Source: CAD feature listing. Evaluate the final solid. Frame: model axes, mm. A direction names the side the tool comes from. Round coordinates to 2 decimals unless told otherwise and drop trailing zeros. Order: outer loops, then holes, each group sorted by start corner. A loop starts at its lowest first (then second) coordinate and runs counter-clockwise, first axis right, second up. Notation, with made-up numbers: (15, 3) - (21, 3) arc R30 ccw to (21, 38) - close; hole circle Ø5 at (-14, -16). An arc over 180 degrees is marked (long way). Return JSON: item names as keys, results as strings. Group by question number.
1) Access query for faces 1 (the flat face through (6, -4, 60)), 2 (the flat face through (7.5, 0, 17)), 3 (the flat face through (-5, 1.1, 39)), 4 (the flat face through (6, -4, 19)), 5 (the flat face through (-6, 4, 39)). Directions: +Z, -Z, +X, -X, +Y, -Y. A direction counts if a zero-diameter tool reaches every point of the face in a straight line with its end or side. Return the directions, or none.
2) Section A-A, the plane y = -5. Return loops of the section in (x, z).
3) Section C-C, the plane y = 0.25. Return loops of the section in (x, z), plus the area to 3 significant figures.
4) Ray query, line 1 (X direction, y = -2.5, z = 72); line 2 (X direction, y = 0, z = 44); line 3 (Z direction, x = 10.25, y = 1.25). Return the intervals inside material, ascending. Write a range as from..to.
5) Section B-B, the plane z = 63. Return loops of the section in (x, y), plus the area to 3 significant figures.
6) Contact query for flat-ended pins moving along their axis: P1, Ø0.9, axis at x = 6, z = 51.5, coming from the -Y side; P2, Ø5, axis at y = 2.5, z = 35, coming from the +X side; P3, Ø1.8, axis at x = 5, z = 35.5, coming from the +Y side. Output: stop coordinate, or through.
7) Section D-D, the plane x = -0.75. Return loops of the section in (y, z), plus the area to 3 significant figures.
8) Mould query, pull axis X, two halves, no side actions, for faces 6 (the flat face through (4.5, 3, 39)), 7 (the flat face through (-6, -4, 39)), 8 (the flat face through (7.5, 0, 61)). Classes: pulls with the +X half, pulls with the -X half, needs draft (parallel to the pull), parting line crosses it, or undercut.
Autodesk Inventor part; units mm, degrees
ref_plane "YZ Plane" through (0, 0, 0) normal (1, 0, 0) x (0, 1, 0)
ref_plane "XZ Plane" through (0, 0, 0) normal (0, 1, 0) x (-1, 0, 0)
ref_plane "XY Plane" through (0, 0, 0) normal (0, 0, 1) x (1, 0, 0)
sketch "Sketch1" plane through (0, 0, 0) normal (0, 0, 1) x (1, 0, 0)
  line L0 (-7.5, 7.5) -> (7.5, 7.5)
  line L1 (7.5, 7.5) -> (7.5, -7.5)
  line L2 (7.5, -7.5) -> (-7.5, -7.5)
  line L3 (-7.5, -7.5) -> (-7.5, 7.5)
  line L4 (-7.5, 7.5) -> (7.5, -7.5) construction
  line L5 (7.5, 7.5) -> (-7.5, -7.5) construction
  line L6 (0, 4.0776) -> (0, -3.6051) construction
  line L7 (-7.5, 4) -> (-4.5, 4)
  line L8 (-4.5, -4) -> (-7.5, -4)
  line L9 (-7.5, -4) -> (-7.5, 4)
  line L10 (-7.5, 4) -> (-4.5, -4) construction
  line L11 (-4.5, 4) -> (-7.5, -4) construction
  line L12 (-6.1, 1.1) -> (-4.5, 1.1)
  line L13 (-2.9, 1.1) -> (-2.9, -1.1)
  line L14 (-4.5, -1.1) -> (-6.1, -1.1)
  line L15 (-6.1, -1.1) -> (-6.1, 1.1)
  line L16 (-6.1, 1.1) -> (-2.9, -1.1) construction
  line L17 (-2.9, 1.1) -> (-6.1, -1.1) construction
  line L18 (7.5, 7.5) -> (-7.5, -7.5) construction
  line L19 (-7.5, 7.5) -> (7.5, -7.5) construction
  line L20 (7.5, 4) -> (4.5, 4)
  line L21 (4.5, -4) -> (7.5, -4)
  line L22 (7.5, 4) -> (4.5, -4) construction
  line L23 (4.5, 4) -> (7.5, -4) construction
  line L24 (6.1, 1.1) -> (4.5, 1.1)
  line L25 (4.5, -1.1) -> (6.1, -1.1)
  line L26 (6.1, -1.1) -> (6.1, 1.1)
  line L27 (6.1, 1.1) -> (2.9, -1.1) construction
  line L28 (2.9, 1.1) -> (6.1, -1.1) construction
  line L29 (4.5, 4) -> (4.5, 1.1)
  line L30 (4.5, -1.1) -> (4.5, -4)
  line L31 (-4.5, 4) -> (-4.5, 1.1)
  line L32 (-4.5, -1.1) -> (-4.5, -4)
  point P0 (0, 0)
  point P1 (-6, 0)
  point P2 (-4.5, 0)
  point P3 (6, 0)
  point P4 (4.5, 0)
  dimension "d0" = 15
  dimension "d1" = 15
  dimension "d2" = 3
  dimension "d3" = 8
  dimension "d6" = 3.2
  dimension "d7" = 2.2
extrude "Extrusion1" add sketch "Sketch1" against normal blind 5
extrude "Extrusion2" add sketch "Sketch1" along normal blind 80 contours L7 L31 L12 L15 L14 L32 L8 L3 | L1 L21 L30 L25 L26 L24 L29 L20
sketch "Sketch2" plane through (4.5, -4, 0) normal (0, -1, 0) x (1, 0, 0)
  line L0 (3, 0) -> (3, 80)
  line L1 (-3, 41) -> (3, 41)
  line L2 (3, 41) -> (3, 39)
  line L3 (3, 39) -> (-3, 39)
  line L4 (-3, 39) -> (-3, 41)
  line L5 (0, 0) -> (0, 80)
  line L6 (-3, 41) -> (3, 39) construction
  line L7 (3, 41) -> (-3, 39) construction
  line L8 (0, 41) -> (0, 39)
  point P0 (-4.5, 0)
  point P1 (0, 40)
  point P2 (3, 41)
  dimension "d12" = 2
extrude "Extrusion3" add sketch "Sketch2" along normal blind 3 contours L3 L5 L1 L0
sketch "Sketch3" plane through (7.5, -7.5, -5) normal (1, 0, 0) x (0, 0, -1)
  line L0 (-44, 0.5) -> (-46, 0.5)
  line L1 (-5, 11.5) -> (-85, 11.5)
  line L2 (-46, 0.5) -> (-44, 0.5)
  line L3 (-44, 0.5) -> (-44, 11.5)
  line L4 (-44, 11.5) -> (-46, 11.5)
  line L5 (-46, 11.5) -> (-46, 0.5)
  point P0 (-5, 7.5)
  dimension "d15" = 2
extrude "Extrusion4" add sketch "Sketch3" along normal blind 3
properties part number "Bracket Lifter_3DPrint"
Geometry check:
{
 "1": {"face 1": "+Z, +X, -X, -Y", "face 2": "-Z, +X, +Y, -Y", "face 3": "+Z", "face 4": "+X, -X, -Y", "face 5": "+Z, +X, -X, +Y"},
 "2": {"outline": "(-7.5, -5) - (7.5, -5) - (7.5, 0) - (-7.5, 0) - close; (4.5, 39) - (10.5, 39) - (10.5, 41) - (4.5, 41) - close"},
 "3": {"outline": "(-7.5, -5) - (7.5, -5) - (7.5, 39) - (10.5, 39) - (10.5, 41) - (7.5, 41) - (7.5, 80) - (6.1, 80) - (6.1, 0) - (-6.1, 0) - (-6.1, 80) - (-7.5, 80) - close", "area": "305 mm2"},
 "4": {"line 1": "-7.5..-4.5, 4.5..7.5", "line 2": "-7.5..-6.1, 6.1..7.5", "line 3": "39..41"},
 "5": {"outline": "(-7.5, -4) - (-4.5, -4) - (-4.5, -1.1) - (-6.1, -1.1) - (-6.1, 1.1) - (-4.5, 1.1) - (-4.5, 4) - (-7.5, 4) - close; (4.5, -4) - (7.5, -4) - (7.5, 4) - (4.5, 4) - (4.5, 1.1) - (6.1, 1.1) - (6.1, -1.1) - (4.5, -1.1) - close", "area": "41.0 mm2"},
 "6": {"P1": "y = -4", "P2": "x = 7.5", "P3": "y = 4"},
 "7": {"outline": "(-7.5, -5) - (7.5, -5) - (7.5, 0) - (-7.5, 0) - close", "area": "75.0 mm2"},
 "8": {"face 6": "undercut", "face 7": "needs draft", "face 8": "pulls with the +X half"}
}
